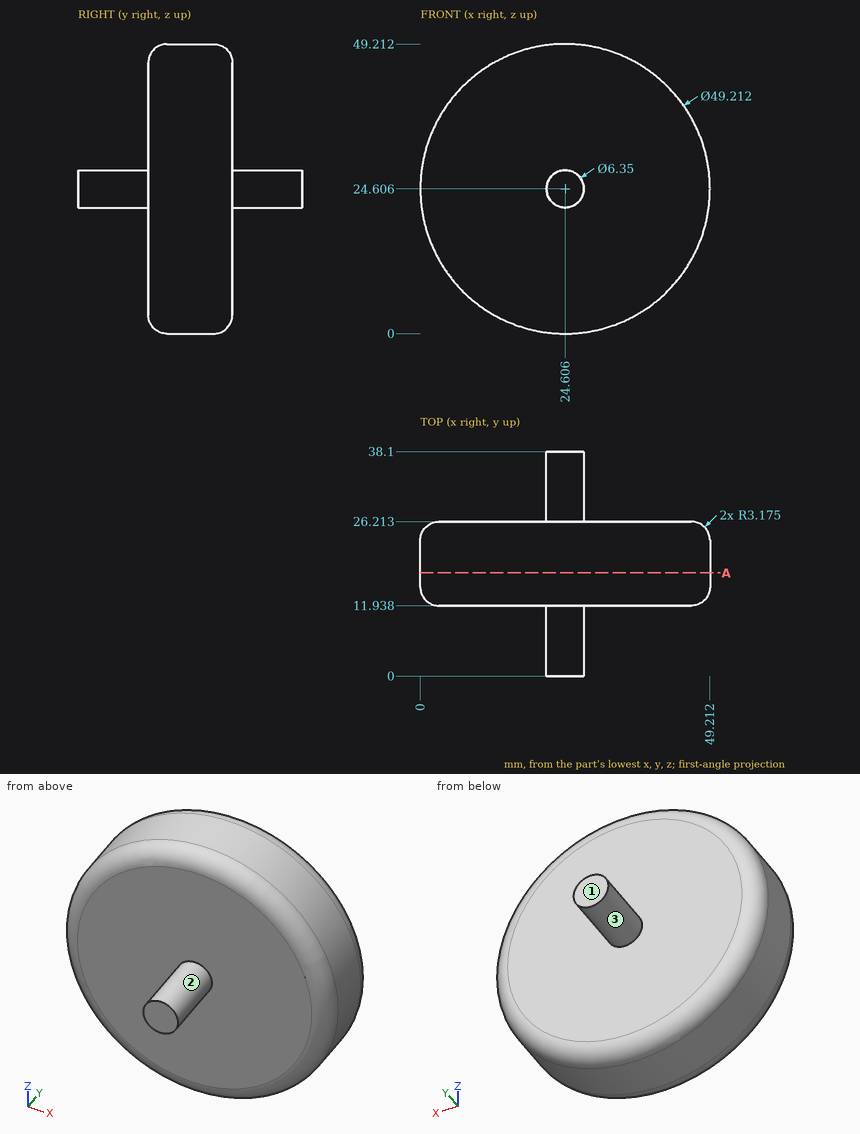
Answer from the drawing. Dimensions are ordinates in mm from the lowest x, y and z of the part. A direction names the side the tool comes from. Round coordinates to 2 decimals unless told otherwise and drop trailing zeros. Write each loop counter-clockwise with the first axis right and the second up, starting at its lowest first coordinate (ties: lowest second). Pieces come first, ordered by that corner, then holes. Notation, with made-up numbers: M 78,25 L 88,25 A30 cw 88,51 Z; hole C -15,-16 d3. An arc over 180 degrees is marked long. Write each question's results on one line, items separated by ' | '. Start each with the question number.
Item 1: Given pin 1 Ø5 at (x, z) = (13.5, 41) entering from -Y; pin 2 Ø10 at (x, z) = (18.5, 18.5) entering from +Y; pin 3 Ø1.5 at (y, z) = (31.5, 21.5) entering from -X; pin 4 Ø2 at (x, y) = (30, 9) entering from +Z, each flat-ended and moving along its own axis, determine where each tip first touches the part or whether it passes through.
Item 2: Which of the six approach directions +Z, -Z, +X, -X, +Y, -Y give full straight-line access (tool end or side, diameter ignored) to the marked faces 1, 2 and 3?
Item 3: Find section A-A on y = 17.5. Write down the section's boundary in (x, z), and give its area (3 significant figures).
Item 4: Straight lines are drawn through the part: probe 1 along Y at (x, z) = (3.5, 26); probe 2 along X at (y, z) = (18, 20.5) (1 decimal); probe 3 along Z at (x, y) = (45, 14.5) (1 decimal). For each, find the intervals that lie inside material, in ascending order.
Answer block:
1) pin 1: stops at y = 11.94 | pin 2: stops at y = 26.21 | pin 3: stops at x = 22.48 | pin 4: passes through
2) face 1: +Z, -Z, +X, -X, +Y | face 2: -Y | face 3: +Y
3) outline: C 24.61,24.61 d49.21 | area: 1,900 mm²
4) probe 1: y = 11.94 to 26.21 | probe 2: x = 0.3 to 48.9 | probe 3: z = 10.9 to 38.3
